Part model, mm, in its own coordinate system. A direction names the side the tool comes from. Round coordinates to 2 decimals unless told otherwise and drop trailing zeros. Write each loop counter-clockwise with the first axis right and the second up, starting at its lowest first coordinate (ties: lowest second). Pieces come first, ordered by that corner, then holes.
```python
from build123d import *

# Parameters (mm, degrees)
SKETCH062_W          = 40
SKETCH062_H          = 100
PAD005_DEPTH         = 18
SKETCH063_R          = 3
SKETCH063_R_2        = 2.5
POCKET035_DEPTH      = 0.001
POCKET035_DEPTH_BACK = 18.001
POCKET041_DEPTH      = 7


with BuildPart() as part:
    # Sketch062 → Pad005 (new body)
    with BuildSketch(Plane.XY):
        Rectangle(SKETCH062_W, SKETCH062_H)
    extrude(amount=PAD005_DEPTH)

    # Sketch063 → Pocket035 (cut, two sides)
    with BuildSketch(Plane.XY) as pocket035_sk:
        with Locations((0, 40)):
            Circle(SKETCH063_R)
        with Locations((0, 20)):
            Circle(SKETCH063_R_2)
        with Locations((0, -40)):
            Circle(SKETCH063_R_2)
    extrude(amount=-POCKET035_DEPTH, mode=Mode.SUBTRACT)
    extrude(pocket035_sk.sketch, amount=POCKET035_DEPTH_BACK, mode=Mode.SUBTRACT)

    # Sketch092 → Pocket041 (cut)
    with BuildSketch(Plane(origin=(0, 40, 18), x_dir=(1, 0, 0), z_dir=(0, 0, 1))):
        Polygon((5.773503, 0), (2.886751, 5), (-2.886751, 5), (-5.773503, 0), (-2.886751, -5), (2.886751, -5), align=None)
    extrude(amount=-POCKET041_DEPTH, mode=Mode.SUBTRACT)


solid = part.part
```
Q1. Cut at B-B on x = 0. Write the cut outline in (y, z).
Values follow:
outline: (-50, 0) - (-42.5, 0) - (-42.5, 18) - (-50, 18) - close; (-37.5, 0) - (17.5, 0) - (17.5, 18) - (-37.5, 18) - close; (22.5, 0) - (37, 0) - (37, 11) - (35, 11) - (35, 18) - (22.5, 18) - close; (43, 0) - (50, 0) - (50, 18) - (45, 18) - (45, 11) - (43, 11) - close
Q2. Mould opens along X. For faces 1 (the flat face through (0, 1, 18)), 2 (the cylindrical face through (-0.54, -42.44, 8.87)), 3 (the flat face through (-20, -1, 9)) say: +X half, -X half, draft (parallel to the pull), parting line (faces both ways), or undercut.
Values follow:
face 1: draft
face 2: undercut
face 3: -X half
Q3. Cut at A-A on y = -40. Write the cut outline in (x, z), plus the area to 3 significant figures.
Values follow:
outline: (-20, 0) - (-2.5, 0) - (-2.5, 18) - (-20, 18) - close; (2.5, 0) - (20, 0) - (20, 18) - (2.5, 18) - close
area: 630 mm2
Q4. Cut at C-C on z = 6.5. Write the cut outline in (x, y).
Values follow:
outline: (-20, -50) - (20, -50) - (20, 50) - (-20, 50) - close; hole circle Ø6 at (0, 40); hole circle Ø5 at (0, -40); hole circle Ø5 at (0, 20)
Q5. Wall check: L1, parallel to Y at x = 0, z = 7; L2, parallel to X at y = 20, z = 10.5; L3, parallel to Z at x = -0.5, y = 44.5. Give the ranges that are in metal, low to high.
Values follow:
L1: y = -50 to -42.5, -37.5 to 17.5, 22.5 to 37, 43 to 50
L2: x = -20 to -2.5, 2.5 to 20
L3: z = 0 to 11
Q6. Drop a flat-ended pin along its axis: pin 1 (5 mm diameter, centred on x = -2, y = 40.5, fed in from +Z). Give the stop position or say it passes through.
Values follow:
pin 1: stops at z = 11
Q7. Which spindle directions (+Z, -Z, +X, -X, +Y, -Y) get a long thin tool onto all of the face, cutting with end or side? Do faces 4 (the flat face through (4.31, 37.465, 14.549)), 5 (the flat face through (0, 50, 9)). Say none if no direction does.
Values follow:
face 4: +Z
face 5: +Z, -Z, +X, -X, +Y
Q8. Cut at D-D on z = 14. Write the cut outline in (x, y).
Values follow:
outline: (-20, -50) - (20, -50) - (20, 50) - (-20, 50) - close; hole (-5.77, 40) - (-2.89, 35) - (2.89, 35) - (5.77, 40) - (2.89, 45) - (-2.89, 45) - close; hole circle Ø5 at (0, -40); hole circle Ø5 at (0, 20)
